from build123d import *

# Parameters (mm, degrees)
F0_R      = 2
F1_DEPTH  = 8
F3_DEPTH  = 185
F5_DEPTH  = 5
F6_R      = 4
F6_R_2    = 2
F7_DEPTH  = 4
F9_DEPTH  = 340
F11_DEPTH = 320
F12_DEPTH = 190
F13_R     = 1.5
F14_DEPTH = 25


with BuildPart() as f1:
    # F0 (on Top) → F1 (new body)
    with BuildSketch(Plane.XY):
        Polygon((248.954638797, 211.431907829), (-84.8453715444, 211.431907829), (-84.8453715444, -69.5673050332), (248.954638797, -69.5673050332), (248.954638797, -32.408092171), align=None)
        with Locations((-44.415361203, -24.153092171)):
            Circle(F0_R, mode=Mode.SUBTRACT)
        with BuildLine():
            Line((-54.4153634839, 33.1772758796), (-54.4153634839, -42.7324894255))
            ThreePointArc((-54.4153634839, -42.7324894255), (-60.3474954333, -48.664621375), (-66.2796273828, -42.7324894255))
            Line((-66.2796273828, -42.7324894255), (-66.2796273828, 33.1772758796))
            ThreePointArc((-66.2796273828, 33.1772758796), (-60.3474954333, 39.109407829), (-54.4153634839, 33.1772758796))
        make_face(mode=Mode.SUBTRACT)
        with BuildLine():
            Line((-19.3557292535, -34.1526738179), (54.9850068476, -34.1526738179))
            ThreePointArc((54.9850068476, -34.1526738179), (63.5648240612, -42.7324878197), (54.9850100594, -51.3123050332))
            Line((54.9850100594, -51.3123050332), (-19.3557260418, -51.3123050332))
            ThreePointArc((-19.3557260418, -51.3123050332), (-27.9355464671, -42.7324910314), (-19.3557292535, -34.1526738179))
        make_face(mode=Mode.SUBTRACT)
        with Locations((80.044638797, -24.153092171)):
            Circle(F0_R, mode=Mode.SUBTRACT)
        with Locations((-44.415361203, 48.236907829)):
            Circle(F0_R, mode=Mode.SUBTRACT)
        with BuildLine():
            ThreePointArc((-34.415361203, 23.1772758796), (-30.0044971271, 33.8260437532), (-19.3557292535, 38.236907829))
            Line((-19.3557292535, 38.236907829), (54.9850068476, 38.236907829))
            ThreePointArc((54.9850068476, 38.236907829), (65.6337747212, 33.8260437532), (70.044638797, 23.1772758796))
            Line((70.044638797, 23.1772758796), (70.044638797, 0.9065397785))
            ThreePointArc((70.044638797, 0.9065397785), (65.6337747212, -9.7422280951), (54.9850068476, -14.153092171))
            Line((54.9850068476, -14.153092171), (-19.3557292535, -14.153092171))
            ThreePointArc((-19.3557292535, -14.153092171), (-30.0044971271, -9.7422280951), (-34.415361203, 0.9065397785))
            Line((-34.415361203, 0.9065397785), (-34.415361203, 23.1772758796))
        make_face(mode=Mode.SUBTRACT)
        with Locations((80.044638797, 48.236907829)):
            Circle(F0_R, mode=Mode.SUBTRACT)
        with BuildLine():
            ThreePointArc((212.4650068476, -34.1526738179), (221.0448240612, -42.7324878197), (212.4650100594, -51.3123050332))
            Line((212.4650100594, -51.3123050332), (105.1042739582, -51.3123050332))
            ThreePointArc((105.1042739582, -51.3123050332), (96.5244567447, -42.7324910314), (105.1042707465, -34.1526738179))
            Line((105.1042707465, -34.1526738179), (212.4650068476, -34.1526738179))
        make_face(mode=Mode.SUBTRACT)
        with Locations((237.524638797, -24.153092171)):
            Circle(F0_R, mode=Mode.SUBTRACT)
        with BuildLine():
            Line((90.044638797, 0.9065397785), (90.044638797, 23.1772758796))
            ThreePointArc((90.044638797, 23.1772758796), (94.4555028729, 33.8260437532), (105.1042707465, 38.236907829))
            Line((105.1042707465, 38.236907829), (212.4650068476, 38.236907829))
            ThreePointArc((212.4650068476, 38.236907829), (223.1137747212, 33.8260437532), (227.524638797, 23.1772758796))
            Line((227.524638797, 23.1772758796), (227.524638797, 0.9065397785))
            ThreePointArc((227.524638797, 0.9065397785), (223.1137747212, -9.7422280951), (212.4650068476, -14.153092171))
            Line((212.4650068476, -14.153092171), (105.1042707465, -14.153092171))
            ThreePointArc((105.1042707465, -14.153092171), (94.4555028729, -9.7422280951), (90.044638797, 0.9065397785))
        make_face(mode=Mode.SUBTRACT)
        with Locations((237.524638797, 48.236907829)):
            Circle(F0_R, mode=Mode.SUBTRACT)
        with BuildLine():
            Line((-54.4153634839, 180.316907829), (-54.4153634839, 63.2965397785))
            ThreePointArc((-54.4153634839, 63.2965397785), (-60.3474954333, 57.364407829), (-66.2796273828, 63.2965397785))
            Line((-66.2796273828, 63.2965397785), (-66.2796273828, 180.316907829))
            ThreePointArc((-66.2796273828, 180.316907829), (-60.3474954333, 186.2490397785), (-54.4153634839, 180.316907829))
        make_face(mode=Mode.SUBTRACT)
        with BuildLine():
            Line((-34.415361203, 73.2965397785), (-34.415361203, 178.1172758796))
            ThreePointArc((-34.415361203, 178.1172758796), (-30.0044971271, 188.7660437532), (-19.3557292535, 193.176907829))
            Line((-19.3557292535, 193.176907829), (54.9850068476, 193.176907829))
            ThreePointArc((54.9850068476, 193.176907829), (65.6337747212, 188.7660437532), (70.044638797, 178.1172758796))
            Line((70.044638797, 178.1172758796), (70.044638797, 73.2965397785))
            ThreePointArc((70.044638797, 73.2965397785), (65.6337747212, 62.6477719049), (54.9850068476, 58.236907829))
            Line((54.9850068476, 58.236907829), (-19.3557292535, 58.236907829))
            ThreePointArc((-19.3557292535, 58.236907829), (-30.0044971271, 62.6477719049), (-34.415361203, 73.2965397785))
        make_face(mode=Mode.SUBTRACT)
        with Locations((-44.415361203, 203.176907829)):
            Circle(F0_R, mode=Mode.SUBTRACT)
        with Locations((80.044638797, 203.176907829)):
            Circle(F0_R, mode=Mode.SUBTRACT)
        with BuildLine():
            ThreePointArc((227.524638797, 73.2965397785), (223.1137747212, 62.6477719049), (212.4650068476, 58.236907829))
            Line((212.4650068476, 58.236907829), (105.1042707465, 58.236907829))
            ThreePointArc((105.1042707465, 58.236907829), (94.4555028729, 62.6477719049), (90.044638797, 73.2965397785))
            Line((90.044638797, 73.2965397785), (90.044638797, 178.1172758796))
            ThreePointArc((90.044638797, 178.1172758796), (94.4555028729, 188.7660437532), (105.1042707465, 193.176907829))
            Line((105.1042707465, 193.176907829), (212.4650068476, 193.176907829))
            Line((212.4650068476, 193.176907829), (212.4650068476, 170.316907829))
            ThreePointArc((212.4650068476, 170.316907829), (223.1137747212, 165.9060437532), (227.524638797, 155.2572758796))
            Line((227.524638797, 155.2572758796), (227.524638797, 73.2965397785))
        make_face(mode=Mode.SUBTRACT)
        with Locations((237.524638797, 180.316907829)):
            Circle(F0_R, mode=Mode.SUBTRACT)
    extrude(amount=F1_DEPTH)

    # F2 (on face) → F3 (join)
    with BuildSketch(Plane.XY.offset(8)):
        Polygon((15.1546284556, 211.431907829), (-84.8453715444, 211.431907829), (-84.8453715444, 71.431907829), (-81.8453715444, 71.431907829), (-81.8453715444, 208.431907829), (15.1546284556, 208.431907829), align=None)
    extrude(amount=F3_DEPTH)

    # F4 (on face) → F5 (cut)
    with BuildSketch(Plane(origin=(-84.8453715444, 0, 0), x_dir=(0, -1, 0), z_dir=(-1, 0, 0))):
        Polygon((-169.016168882, 40), (-201.431907829, 143.5533241114), (-201.431907829, 40), align=None)
        Polygon((-71.431907829, 193), (-206.431907829, 193), (-158.5376649213, 40), (-71.431907829, 40), align=None)
    extrude(amount=-F5_DEPTH, mode=Mode.SUBTRACT)

    # F6 (on face) → F7 (join)
    with BuildSketch(Plane.XY.offset(8)):
        with Locations((-44.415361203, 48.236907829)):
            Circle(F6_R)
        with Locations((-44.415361203, 48.236907829)):
            Circle(F6_R_2, mode=Mode.SUBTRACT)
        with Locations((-44.415361203, -24.153092171)):
            Circle(F6_R)
        with Locations((-44.415361203, -24.153092171)):
            Circle(F6_R_2, mode=Mode.SUBTRACT)
    extrude(amount=F7_DEPTH)

    # F8 (on face) → F9 (cut)
    with BuildSketch(Plane.YZ.offset(248.954638797)):
        Polygon((57.7434247732, 4), (37.7434247732, 4), (37.7434247732, 0), (211.431907829, 0), (211.431907829, 8), (57.7434247732, 8), align=None)
    extrude(amount=-F9_DEPTH, mode=Mode.SUBTRACT)

    # F10 (on face) → F11 (cut)
    with BuildSketch(Plane(origin=(0, 211.431907829, 0), x_dir=(-1, 0, 0), z_dir=(0, 1, 0))):
        Polygon((-89.7116868198, 4), (-69.7116868198, 4), (-69.7116868198, 8), (-270.7538604736, 8), (-270.7538604736, -15.3804672882), (-89.7116868198, 0), align=None)
    extrude(amount=-F11_DEPTH, mode=Mode.SUBTRACT)

    # F12 (cut): a face of the model
    f12_faces = [f1.faces().sort_by_distance(p)[0] for p in [
        (13.4341634022, 209.931907829, 8),
    ]]
    extrude(f12_faces, amount=-F12_DEPTH, mode=Mode.SUBTRACT)

    # F13 (on face) → F14 (cut)
    with BuildSketch(Plane.XY.offset(8)):
        with Locations((28.1716429389, -66.5673050332)):
            Circle(F13_R)
        with Locations((-48.4283570611, -66.5673050332)):
            Circle(F13_R)
    extrude(amount=-F14_DEPTH, mode=Mode.SUBTRACT)


solid = f1.part
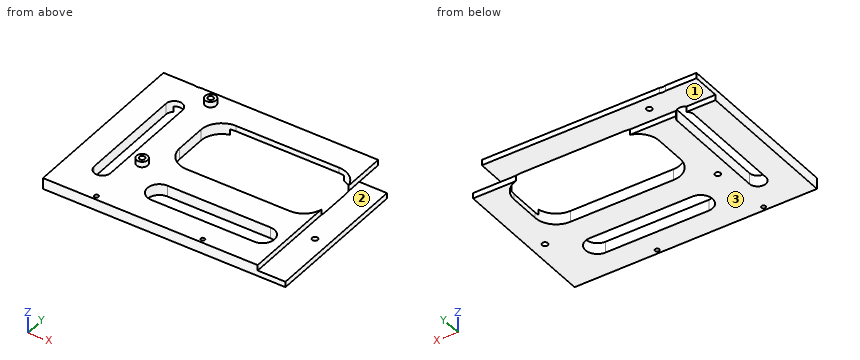
Check sheet for the modelled part. Datum: model origin and axes. Units: mm. Face numbers are marked on the shaded views. A direction names the side the tool comes from. Give positions to 0.01 mm unless a question says otherwise; leave off trailing zeros. Write each loop counter-clockwise with the first axis right and the second up, starting at its lowest first coordinate (ties: lowest second). Pieces come first, ordered by that corner, then holes. Notation, with made-up numbers: (26, -30) -> (67, -30) arc R19 ccw to (67, -16) -> close; hole circle Ø11 at (8, 8.5). An arc over 180 degrees is marked (long way). Use one line per item in the form item = value. Start each with the question number.
1. Section check B-B (y = 3). Record the cut outline in (x, z).
2. Access from +Z, -Z, +X, -X, +Y, -Y to the whole of each face (thin tool, end or side, straight path). Record for the marked faces 1, 2 and 3.
3. Section check A-A (x = 49). Record the cut outline in (y, z), and give its area (3 significant figures).
4. Go/stop test with flat-tipped pins: P1, Ø3, axis at y = 49.5, z = 6.5, coming from the +X side; P2, Ø10, axis at x = 4, y = 45.5, coming from the -Z side; P3, Ø2, axis at x = 13.5, y = -24.5, coming from the +Z side. Record where each tip stops, or that it passes through.
5. Thickness scan on line 1 along Y through (x, z) = (38.5, 4.25); line 2 along Y through (x, z) = (27, 2.25); line 3 along X through (y, z) = (-11, 1). Record the ranges inside material, lowest first. Write a range as from..to.
Conclusion:
q1.outline = (-84.85, 0) -> (-66.28, 0) -> (-66.28, 8) -> (-84.85, 8) -> close; (-54.42, 0) -> (-34.42, 0) -> (-34.42, 8) -> (-54.42, 8) -> close; (70.04, 0) -> (89.71, 0) -> (89.71, 4) -> (70.04, 4) -> close
q2.face_1 = -Z, +X, -X, +Y
q2.face_2 = +Z, +X, +Y, -Y
q2.face_3 = -Z, +X, -X, +Y, -Y
q3.outline = (-69.57, 0) -> (-51.31, 0) -> (-51.31, 8) -> (-69.57, 8) -> close; (-34.15, 0) -> (-14.15, 0) -> (-14.15, 8) -> (-34.15, 8) -> close; (38.24, 4) -> (57.74, 4) -> (57.74, 8) -> (38.24, 8) -> close
q3.area = 384 mm²
q4.P1 = 69.71
q4.P2 = 4
q4.P3 = 8
q5.line_1 = -69.57..-51.31, -34.15..-14.15, 38.24..57.74
q5.line_2 = -69.57..-67.5, -65.63..-51.31, -34.15..-14.15
q5.line_3 = -84.85..-66.28, -54.42..-28.58, 64.21..89.71
